Could you check a few things on this model? Use its own coordinates, in mm. A direction names the side the tool comes from. Coordinates: 2 decimals unless noted, no trailing zeros. Loops run counter-clockwise (first coordinate to the right, second up) from the corner with the lowest first, then second, coordinate; pieces in that order, holes last. Notation, with made-up numbers: (50.25, 58.5) -> (61.25, 58.5) arc R26 ccw to (61.25, 78.5) -> close; hole circle Ø11 at (33.5, 51). An arc over 180 degrees is marked (long way). One line per question, with ' | ' between items. Start each with the question number.
(1) Suppose I cut it at B-B (z = 71.5). Please give me the cut outline in (x, y).
(2) Suppose I cut it at C-C (x = 37). Please give me the cut outline in (y, z).
(3) I'm going to push flat-ended pins straight in: pin 1 Ø9.5 at (x, z) = (-36, 47) entering from +Y; pin 2 Ø15 at (x, z) = (42.5, 33) entering from +Y; pin 3 Ø10.5 at (x, y) = (13, -4.5) entering from -Z. Where does each tip first touch, or does it pass through?
(4) Suppose I cut it at A-A (y = 7). Please give me the cut outline in (x, z).
(5) If we mould it in two halves opening along Y, with no side actions, what happens to faces 5 (the face through (-38, 0, 32)), 6 (the face through (3, -9.414, 107)), 7 (the face through (35.38, 7, 40))? For each: pulls with the +Y half, pulls with the -Y half, needs draft (parallel to the pull), parting line crosses it, or undercut.
(6) If I drill on line 1 along X through (y, z) = (-6, 49); line 2 along Y through (x, z) = (42, 111); line 3 along Z through (x, y) = (6, -3), over which ranges is the centre line in solid material (lowest first)?
(7) Suppose I cut it at D-D (z = 45.5). Please give me the cut outline in (x, y).
(8) Which directions (+Z, -Z, +X, -X, +Y, -Y) give clear straight access to the entire face, cutting with the end or side of a thin tool? Please do faces 1 (the face through (45, 0, 32)), 2 (the face through (4, -5, 127)), 3 (the face through (3, 0, 110)), 4 (the face through (-28.12, 7, 39)).
```python
from build123d import *

# Parameters (mm, degrees)
F1_W     = 19.05
F1_H     = 19.05
F0_W     = 19.05
F0_H     = 19.05
F0_H_2   = 25.4
F0_W_2   = 63.5
F0_H_3   = 63.5
F4_DEPTH = 9.4144362956


with BuildPart() as f2:
    # F1 (on Top) → F2 section 0
    with BuildSketch(Plane.XY):
        with Locations((44.9054742098, 22.225)):
            Rectangle(F1_W, F1_H)
    # F0 (on Front) → F2 section 1
    with BuildSketch(Plane.XZ):
        with Locations((44.9054742098, 73.025)):
            Rectangle(F0_W, F0_H)
    loft()



with BuildPart() as f3:
    # F1 (on Top) → F3 section 0
    with BuildSketch(Plane.XY):
        with Locations((-37.6445257902, 22.225)):
            Rectangle(F1_W, F1_H)
    # F0 (on Front) → F3 section 1
    with BuildSketch(Plane.XZ):
        with Locations((-37.6445257902, 73.025)):
            Rectangle(F0_W, F0_H)
    loft()


with BuildPart() as f2_1:
    add(f2.part)

    add(f3.part)  # F4 merges F3
    # F0 (on Front) → F4 (join)
    with BuildSketch(Plane.XZ):
        with Locations((-37.6445257902, 92.075)):
            Rectangle(F0_W, F0_H)
        with Locations((-37.6445257902, 114.3)):
            Rectangle(F0_W, F0_H_2)
        with Locations((3.6304742098, 114.3)):
            Rectangle(F0_W_2, F0_H_2)
        with Locations((44.9054742098, 114.3)):
            Rectangle(F0_W, F0_H_2)
        with Locations((44.9054742098, 92.075)):
            Rectangle(F0_W, F0_H)
        with Locations((-37.6445257902, 31.75)):
            Rectangle(F0_W, F0_H_3)
        with Locations((-37.6445257902, 73.025)):
            Rectangle(F0_W, F0_H)
        with Locations((44.9054742098, 31.75)):
            Rectangle(F0_W, F0_H_3)
        with Locations((44.9054742098, 73.025)):
            Rectangle(F0_W, F0_H)
    extrude(amount=F4_DEPTH)


solid = f2_1.part
```
Checks:
1) outline: (-47.17, -9.41) -> (-28.12, -9.41) -> (-28.12, 4.25) -> (-47.17, 4.25) -> close; (35.38, -9.41) -> (54.43, -9.41) -> (54.43, 4.25) -> (35.38, 4.25) -> close
2) outline: (-9.41, 0) -> (0, 0) -> (0, 63.5) -> (12.7, 0) -> (31.75, 0) -> (0, 82.55) -> (0, 127) -> (-9.41, 127) -> close
3) pin 1: stops at y = 15.5 | pin 2: stops at y = 21.94 | pin 3: stops at z = 101.6
4) outline: (-47.17, 28.5) -> (-28.12, 28.5) -> (-28.12, 64.35) -> (-47.17, 64.35) -> close; (35.38, 28.5) -> (54.43, 28.5) -> (54.43, 64.35) -> (35.38, 64.35) -> close
5) face 5: undercut | face 6: pulls with the -Y half | face 7: needs draft
6) line 1: x = -47.17 to -28.12, 35.38 to 54.43 | line 2: y = -9.41 to 0 | line 3: z = 101.6 to 127
7) outline: (-47.17, -9.41) -> (-28.12, -9.41) -> (-28.12, 0) -> (-47.17, 0) -> close; (-47.17, 3.6) -> (-28.12, 3.6) -> (-28.12, 14.25) -> (-47.17, 14.25) -> close; (35.38, -9.41) -> (54.43, -9.41) -> (54.43, 0) -> (35.38, 0) -> close; (35.38, 3.6) -> (54.43, 3.6) -> (54.43, 14.25) -> (35.38, 14.25) -> close
8) face 1: -Z, +X, -X | face 2: +Z, +X, -X, +Y, -Y | face 3: +Z, +X, -X, +Y | face 4: -Z, +Y, -Y
